Autodesk Fusion 360 part; units mm, degrees
sketch "Esquisse2" plane through (0, 0, 0) normal (0, 0, 1) x (1, 0, 0)
  line L0 (0, 0) -> (33.5, 0)
  line L1 (0, 0) -> (-2.6172, 59.9429)
  line L2 (0, 0) -> (60, 0) construction
  line L3 (33.5, 0) -> (32.7156, 8.9658)
  line L4 (33.5, 0) -> (42.4658, 0) construction
  line L5 (32.7156, 8.9658) -> (40.0032, 10.2507)
  line L6 (32.7156, 8.9658) -> (40.1156, 8.9658) construction
  line L7 (40.0032, 10.2507) -> (36.8897, 61.1556)
  line L8 (40.0032, 10.2507) -> (91.0032, 10.2507) construction
  line L9 (36.8897, 61.1556) -> (-2.6172, 59.9429)
  dimension "d13" = 33.5
  dimension "d14" = 92.5
  dimension "d15" = 60
  dimension "d16" = 95
  dimension "d17" = 9
  dimension "d18" = 10
  dimension "d19" = 7.4
  dimension "d20" = 93.5
  dimension "d21" = 51
sketch "Esquisse3" plane through (0, 0, 0) normal (0, 0, 1) x (1, 0, 0)
  line L0 (0, 0) -> (-5, 0) construction
  line L1 (-5, 0) -> (-5, -5) construction
  line L2 (-5, -5) -> (0, -5) construction
  line L3 (0, -5) -> (0, 0) construction
  line L4 (-5, -5) -> (38.5, -5)
  line L5 (-5, -5) -> (-7.8353, 59.9381)
  line L6 (-5, -5) -> (65, -5) construction
  line L7 (38.5, -5) -> (37.7156, 3.9658)
  line L8 (38.5, -5) -> (47.4658, -5) construction
  line L9 (37.7156, 3.9658) -> (45.0032, 5.2507)
  line L10 (37.7156, 3.9658) -> (45.1156, 3.9658) construction
  line L11 (45.0032, 5.2507) -> (41.5845, 61.1463)
  line L12 (45.0032, 5.2507) -> (106.0032, 5.2507) construction
  line L13 (-7.8353, 59.9381) -> (41.5845, 61.1463)
  dimension "d22" = 5
  dimension "d23" = 5
  dimension "d24" = 43.5
  dimension "d25" = 92.5
  dimension "d26" = 65
  dimension "d27" = 95
  dimension "d28" = 9
  dimension "d29" = 10
  dimension "d30" = 7.4
  dimension "d31" = 93.5
  dimension "d32" = 56
extrude "Extrusion1" add sketch "Esquisse3" along normal blind 35
extrude "Extrusion2" cut sketch "Esquisse2" along normal blind 35
extrude "Extrusion3" cut 1 faces at (10.4829, 60.345, 23.3333) along direction (-0.030682, 0.999529, 0) blind 10
ref_plane "Plan de construction1" through (36.8973, 61.0317, 35) normal (-0.9981, -0.061, 0) x (0.061, -0.9981, 0)
sketch "Esquisse4" plane through (36.8973, 61.0317, 35) normal (-0.9981, -0.061, 0) x (0.061, -0.9981, 0)
  line L0 (0, 0) -> (35, 0) construction
  line L1 (35, 0) -> (35, -17.5) construction
  line L2 (35, -17.5) -> (0, -17.5) construction
  line L3 (0, -17.5) -> (0, 0) construction
  circle A0 centre (35, -17.5) radius 3.8
  dimension "d41" = 35
  dimension "d42" = 17.5
  dimension "d43" = 7.6
ref_plane "Plan de construction2" through (44.0247, 26.4022, 17.5) normal (-0.9981, -0.061, 0) x (0.061, -0.9981, 0)
sketch "Esquisse5" plane through (44.0247, 26.4022, 17.5) normal (-0.9981, -0.061, 0) x (0.061, -0.9981, 0)
  circle A0 centre (0, 0) radius 2
  dimension "d45" = 4
loft "Lissage1" cut profiles "Esquisse5", "Esquisse4" section 1 section 2
ref_plane "Plan de construction3" through (-7.8353, 59.9381, 35) normal (-0.999, -0.0436, 0) x (0.0436, -0.999, 0)
sketch "Esquisse6" plane through (-7.8353, 59.9381, 35) normal (-0.999, -0.0436, 0) x (0.0436, -0.999, 0)
  line L0 (0, 0) -> (35, 0) construction
  line L1 (35, 0) -> (35, -17.5) construction
  line L2 (35, -17.5) -> (0, -17.5) construction
  line L3 (0, -17.5) -> (0, 0) construction
  circle A0 centre (35, -17.5) radius 3.5
  dimension "d46" = 35
  dimension "d47" = 17.5
  dimension "d48" = 7
extrude "Extrusion4" cut sketch "Esquisse6" against normal blind 10
equation "height = 60 mm"
equation "bottomWidth = 33.5 mm"
equation "edgeHeight = 9 mm"
equation "edgeWidth = 7.4 mm"
equation "thickness = 5 mm"
equation "screwHoleDiameter = 4 mm"
equation "screwHoleBevel = 7.6 mm"
equation "screwDriverHoleDiameter = 7 mm"
equation "angle1 = 92.5 deg"
equation "angle2 = 95 deg"
equation "angle3 = 10 deg"
equation "angle4 = 93.5 deg"
equation "d13 = bottomWidth"
equation "d14 = angle1"
equation "d15 = height"
equation "d16 = angle2"
equation "d18 = angle3"
equation "d19 = edgeWidth"
equation "d20 = angle4"
equation "d21 = height - edgeHeight"
equation "d22 = thickness"
equation "d23 = thickness"
equation "d24 = bottomWidth + ( 2 * thickness )"
equation "d25 = angle1"
equation "d26 = height + thickness"
equation "d27 = angle2"
equation "d28 = edgeHeight"
equation "d29 = angle3"
equation "d30 = edgeWidth"
equation "d31 = angle4"
equation "d32 = height - edgeHeight + thickness"
equation "d33 = width"
equation "width = 35 mm"
equation "d36 = width"
equation "screwHoleHeight = 30 mm"
equation "d41 = height + thickness - screwHoleHeight"
equation "d42 = width / 2"
equation "d43 = screwHoleBevel"
equation "d45 = screwHoleDiameter"
equation "d46 = height + thickness - screwHoleHeight"
equation "d47 = width / 2"
equation "d48 = screwDriverHoleDiameter"
equation "d49 = -thickness * 2"
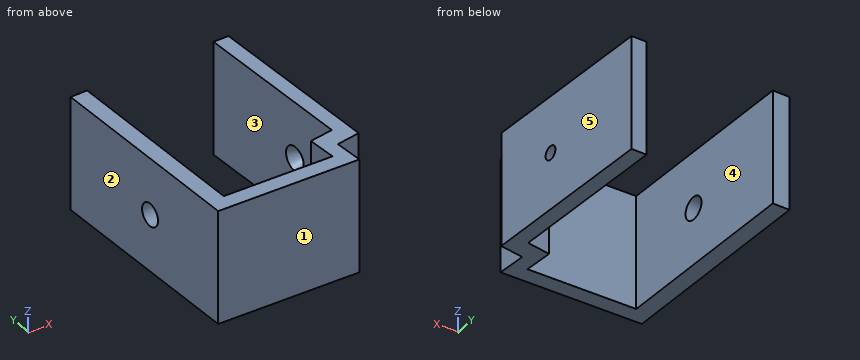
Could you check a few things on this model? Use its own coordinates, in mm. Face numbers are marked on the shaded views. A direction names the side the tool comes from. Coordinates: 2 decimals unless noted, no trailing zeros. Loops run counter-clockwise (first coordinate to the right, second up) from the corner with the lowest first, then second, coordinate; pieces in that order, holes last.
1) Imagine slicing it at C-C (x = 13). List the corners of the cut face in (y, z) for me, and give its area (3 significant figures).
Reported:
outline: (-5, 0) - (0, 0) - (0, 35) - (-5, 35) - close
area: 175 mm2
2) Imagine slicing it at A-A (z = 11.5). List the corners of the cut face in (x, y) for me, and give its area (3 significant figures).
Reported:
outline: (-7.84, 59.94) - (-5, -5) - (38.5, -5) - (37.72, 3.97) - (45, 5.25) - (41.58, 61.15) - (36.9, 61.03) - (40, 10.25) - (32.72, 8.97) - (33.5, 0) - (0, 0) - (-2.62, 59.94) - (-2.62, 60.07) - close
area: 853 mm2
3) Thinking about a two-plate mould opening in X: for the marked faces 1, 2 and 3, which applies, released by +X, released by -X, zero draft, split by the parting line, or undercut?
Reported:
face 1: zero draft
face 2: released by -X
face 3: undercut
4) Which directions (+Z, -Z, +X, -X, +Y, -Y) give clear straight access to the entire face, cutting with the end or side of a thin tool? Please do the marked faces 4 and 5.
Reported:
face 4: +Z, -Z, +Y
face 5: +Z, -Z, +X, +Y
5) Imagine slicing it at B-B (y = 39). List the corners of the cut face in (x, z) for me, and give its area (3 significant figures).
Reported:
outline: (-6.92, 0) - (-1.7, 0) - (-1.7, 35) - (-6.92, 35) - close; (38.24, 0) - (42.94, 0) - (42.94, 35) - (38.24, 35) - close
area: 347 mm2
6) Please list where these lines run through material, in increasing order: line 1 along Y through (x, z) = (25, 17.5); line 2 along X through (y, z) = (46.5, 22); line 3 along X through (y, z) = (33.5, 31).
Reported:
line 1: y = -5 to 0
line 2: x = -7.25 to -2.03, 37.79 to 42.48
line 3: x = -6.68 to -1.46, 38.58 to 43.28
7) Will these pins go through, and if not, where does the flat tip stop? pin 1 Ø1 at (y, z) = (15, 18.5) entering from +X; pin 2 Ø2 at (x, y) = (1, 24) entering from +Z; pin 3 Ø1.5 at (y, z) = (24, 26) entering from +X; pin 4 Ø3 at (x, z) = (7.5, 3.5) entering from +Y.
Reported:
pin 1: stops at x = 44.44
pin 2: passes through
pin 3: stops at x = 43.9
pin 4: stops at y = 0
8) Imagine slicing it at D-D (x = 35.5). List the corners of the cut face in (y, z) for me.
Reported:
outline: (-5, 0) - (9.46, 0) - (9.46, 35) - (-5, 35) - close
